Work out the finished part from the listing and answer in its coordinate system (mm). Face numbers are marked on the shaded views. A direction names the side the tool comes from. Give positions to 0.01 mm unless a question says otherwise; leave off trailing zeros. Write each loop counter-clockwise with the first axis right and the second up, starting at its lowest first coordinate (ties: lowest second). Pieces come first, ordered by that corner, then holes. Notation, with made-up numbers: (44, 13.25) - (80, 13.25) arc R20 ccw to (80, 38.25) - close; hole circle Ø5 at (-35.75, -7). An arc over 180 degrees is marked (long way). Write item = value, one per line.
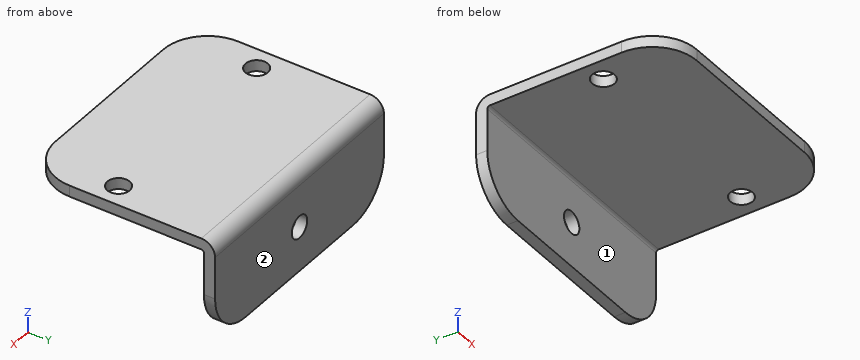
from build123d import *

# Parameters (mm, degrees)
BASE_FLANGE1_DEPTH = 34.925
SKETCH6_R          = 3.175
CUT_EXTRUDE1_DEPTH = 68.947967225
FILLET1_R          = 12.7
SKETCH7_R          = 3.175
CUT_EXTRUDE2_DEPTH = 70.124642856


# Sheet-metal steps are written as plain solids
with BuildPart() as part:
    # Sketch1 → Base-Flange1 (new, symmetric)
    with BuildSketch(Plane(origin=(0, 0, 0), x_dir=(0, 0, -1), z_dir=(1, 0, 0))):
        with BuildLine():
            Line((25.4, 0), (0.7366, 0))
            ThreePointArc((0.7366, 0), (0.215745145, -0.215745145), (0, -0.7366))
            Line((0, -0.7366), (0, -50.8))
            Line((0, -50.8), (-3.175, -50.8))
            Line((-3.175, -50.8), (-3.175, -0.7366))
            ThreePointArc((-3.175, -0.7366), (-2.029318885, 2.029318885), (0.7366, 3.175))
            Line((0.7366, 3.175), (25.4, 3.175))
            Line((25.4, 3.175), (25.4, 0))
        make_face()
    extrude(amount=BASE_FLANGE1_DEPTH, both=True)

    # Sketch6 → Cut-Extrude1 (cut, through all)
    with BuildSketch(Plane.XY.offset(3.175)):
        with Locations((-28.575, -28.575)):
            Circle(SKETCH6_R)
        with Locations((28.575, -28.575)):
            Circle(SKETCH6_R)
    extrude(amount=-CUT_EXTRUDE1_DEPTH, mode=Mode.SUBTRACT)

    # Fillet1
    fillet1_edges = [part.edges().sort_by_distance(p)[0] for p in [
        (34.925, 1.5875, -25.4),
        (34.925, -50.8, 1.5875),
        (-34.925, 1.5875, -25.4),
        (-34.925, -50.8, 1.5875),
    ]]
    fillet(fillet1_edges, radius=FILLET1_R)

    # Sketch7 → Cut-Extrude2 (cut, through all)
    with BuildSketch(Plane(origin=(0, 3.175, 0), x_dir=(1, 0, 0), z_dir=(0, 1, 0))):
        with Locations(Location((0, 12.7, 0), (0, 0, 270))):
            Circle(SKETCH7_R)
    extrude(amount=-CUT_EXTRUDE2_DEPTH, mode=Mode.SUBTRACT)


solid = part.part
1. A tool of negligible diameter and unlimited length cuts with its end or side. For the marked faces 1 and 2, from which of +Z, -Z, +X, -X, +Y, -Y can it reach the whole face along a straight path? Write none if from no direction.
Solution:
face_1 = -Z, +X, -X, -Y
face_2 = +Z, -Z, +X, -X, +Y
2. Given pin 1 (6 mm diameter, centred on x = 15.5, y = -40, fed in from -Z); pin 2 (8 mm diameter, centred on x = -5.5, z = -4.5, fed in from -Y); pin 3 (5 mm diameter, centred on x = 28.575, y = -28.575, fed in from -Z), each flat-ended and moving along its own axis, determine where each tip first touches the part or whether it passes through.
Solution:
pin_1 = 0
pin_2 = -0.04
pin_3 = through
3. Find section C-C, the plane z = -6.5. Give the vertices of the cut face in (x, y) (3 decimals), then the cut area to 3 significant figures.
Solution:
outline = (-34.925, 0) - (34.925, 0) - (34.925, 3.175) - (-34.925, 3.175) - close
area = 222 mm^2
4. Find section B-B, the plane x = 18. Give the vertices of the cut face in (y, z) (3 decimals).
Solution:
outline = (-50.8, 0) - (-0.737, 0) arc R0.737 cw to (0, -0.737) - (0, -25.4) - (3.175, -25.4) - (3.175, -0.737) arc R3.912 ccw to (-0.737, 3.175) - (-50.8, 3.175) - close
5. Find section A-A, the plane x = 0. Give the vertices of the cut face in (y, z) (3 decimals).
Solution:
outline = (-50.8, 0) - (-0.737, 0) arc R0.737 cw to (0, -0.737) - (0, -9.525) - (3.175, -9.525) - (3.175, -0.737) arc R3.912 ccw to (-0.737, 3.175) - (-50.8, 3.175) - close; (0, -25.4) - (3.175, -25.4) - (3.175, -15.875) - (0, -15.875) - close
6. Straight lines are drawn through the part: line 1 (X direction, y = 2.05, z = -12.7) (3 decimals); line 2 (Y direction, x = 19, z = -8.5) (3 decimals). For each, find the intervals that lie inside material, in ascending order.
Solution:
line_1 = -34.925 to -3.175, 3.175 to 34.925
line_2 = 0 to 3.175
